from build123d import *

# Parameters (mm, degrees)
SKETCH1_W           = 70
SKETCH1_H           = 43
SKETCH1_R           = 16.5
SKETCH1_R_2         = 2.25
SKETCH1_R_3         = 2
BOSS_EXTRUDE1_DEPTH = 3


with BuildPart() as part:
    # Sketch1 → Boss-Extrude1 (new body)
    with BuildSketch(Plane(origin=(0, 0, 0), x_dir=(1, 0, 0), z_dir=(0, 1, 0))):
        Rectangle(SKETCH1_W, SKETCH1_H)
        with Locations(Location((-15, 0, 0), (0, 0, 270))):
            Circle(SKETCH1_R, mode=Mode.SUBTRACT)
        with Locations(Location((-1.46, 14.58, 0), (0, 0, 270))):
            Circle(SKETCH1_R_2, mode=Mode.SUBTRACT)
        with Locations(Location((-28.37, -14.7, 0), (0, 0, 270))):
            Circle(SKETCH1_R_2, mode=Mode.SUBTRACT)
        with Locations(Location((25, 8, 0), (0, 0, 270))):
            Circle(SKETCH1_R_3, mode=Mode.SUBTRACT)
        with Locations(Location((25, -8, 0), (0, 0, 270))):
            Circle(SKETCH1_R_3, mode=Mode.SUBTRACT)
    extrude(amount=BOSS_EXTRUDE1_DEPTH)


solid = part.part
Here's how the part is built. I have some questions about the finished solid (model axes, mm). Coordinates: 2 decimals unless noted, no trailing zeros. Write each loop counter-clockwise with the first axis right and the second up, starting at its lowest first coordinate (ties: lowest second). Pieces come first, ordered by that corner, then holes. Notation, with made-up numbers: (-8, 68) - (23, 68) arc R14 cw to (23, 85) - close; hole circle Ø2 at (-30, 48.5). An arc over 180 degrees is marked (long way). Use one line per item in the form item = value.
1) Thinking about a two-plate mould opening in X: for faces 1 (the flat face through (35, 1, 0)), 2 (the cylindrical face through (23.8, 1.5, -9.6)), 3 (the flat face through (7, 3, 0)), which applies, released by +X, released by -X, zero draft, split by the parting line, or undercut?
Solved:
face_1 = released by +X
face_2 = undercut
face_3 = zero draft
2) Suppose I cut it at A-A, the plane x = 25. Write out the boundary of the cut face in (y, z).
Solved:
outline = (0, -21.5) - (3, -21.5) - (3, -10) - (0, -10) - close; (0, -6) - (3, -6) - (3, 6) - (0, 6) - close; (0, 10) - (3, 10) - (3, 21.5) - (0, 21.5) - close
3) I'm going to push a flat-ended pin straight in: P1, Ø2.5, axis at x = -28.37, z = 14.7, coming from the -Y side. Where does the tip first touch, or does it pass through?
Solved:
P1 = through
4) Suppose I cut it at C-C, the plane x = -15. Write out the boundary of the cut face in (y, z), plus the area to 3 significant figures.
Solved:
outline = (0, -21.5) - (3, -21.5) - (3, -16.5) - (0, -16.5) - close; (0, 16.5) - (3, 16.5) - (3, 21.5) - (0, 21.5) - close
area = 30.0 mm2
5) Suppose I cut it at B-B, the plane z = 0. Write out the boundary of the cut face in (x, y), plus the area to 3 significant figures.
Solved:
outline = (-35, 0) - (-31.5, 0) - (-31.5, 3) - (-35, 3) - close; (1.5, 0) - (35, 0) - (35, 3) - (1.5, 3) - close
area = 111 mm2
6) I need wall thicknesses on line 1 (X direction, y = 1.35, z = 0); line 2 (Z direction, x = -28.5, y = 0.2); line 3 (X direction, y = 2.6, z = 14.5). Which ranges of each line are inside material? Lowest first, please.
Solved:
line_1 = -35 to -31.5, 1.5 to 35
line_2 = -21.5 to -9.49, 9.49 to 12.45, 16.95 to 21.5
line_3 = -35 to -30.61, -26.13 to -22.87, -7.13 to 35
7) Suppose I cut it at D-D, the plane z = 8. Write out the boundary of the cut face in (x, y).
Solved:
outline = (-35, 0) - (-29.43, 0) - (-29.43, 3) - (-35, 3) - close; (-0.57, 0) - (23, 0) - (23, 3) - (-0.57, 3) - close; (27, 0) - (35, 0) - (35, 3) - (27, 3) - close
